Geometry: see drawing. Coordinates: mm, zero at the bounding-box minimum. A direction names the side the tool comes from. Round coordinates to 2 decimals unless told otherwise and drop trailing zeros. Loops run counter-clockwise (first coordinate to the right, second up) from the corner with the lowest first, then second, coordinate; pieces in that order, holes last. Notation, with made-up numbers: (9, 48) -> (62, 48) arc R20 ccw to (62, 76) -> close; hole circle Ø5 at (61, 60). An arc over 180 degrees is marked (long way). Write item = value, one per line.
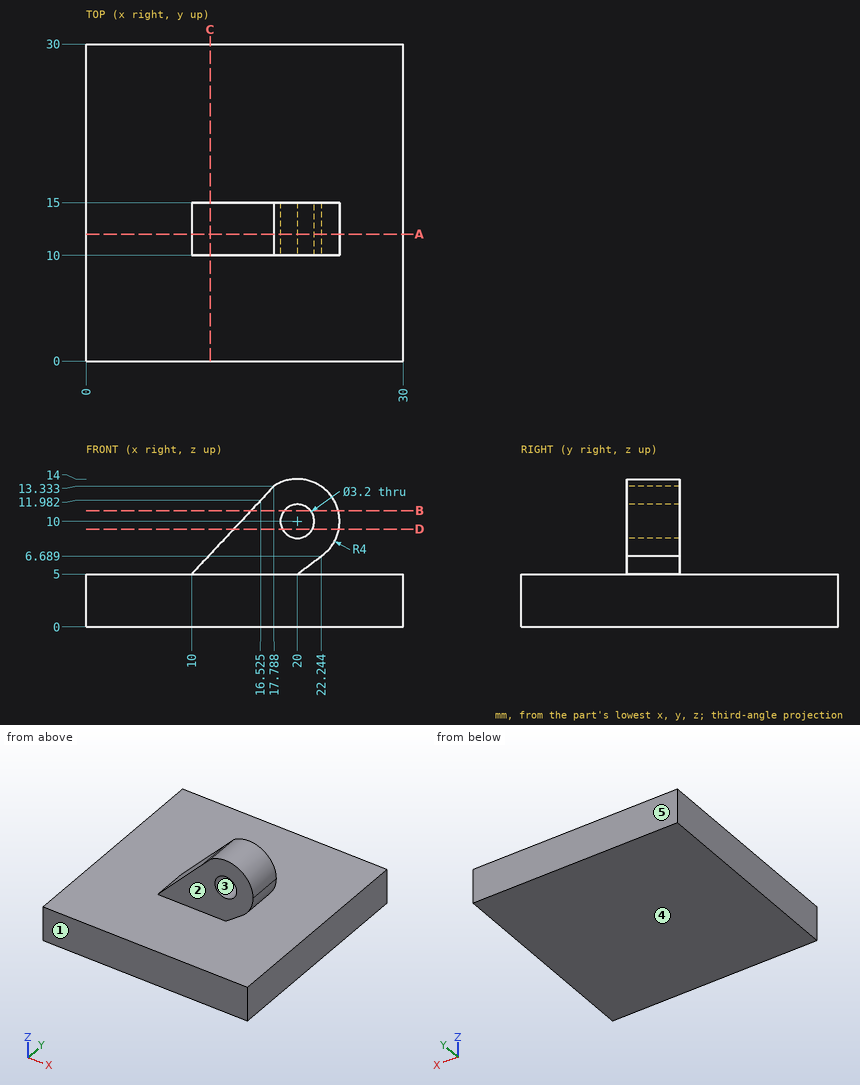
1. Section query B-B (z = 11). Return the cut outline in (x, y).
Evaluation:
outline = (15.61, 10) -> (18.75, 10) -> (18.75, 15) -> (15.61, 15) -> close; (21.25, 10) -> (23.87, 10) -> (23.87, 15) -> (21.25, 15) -> close
2. Section query A-A (y = 12). Return the cut outline in (x, z) (1 decimal).
Evaluation:
outline = (0, 0) -> (30, 0) -> (30, 5) -> (20, 5) -> (22.2, 6.7) arc R4 ccw to (24, 10) arc R4 ccw to (17.8, 13.3) -> (10, 5) -> (0, 5) -> close; hole circle Ø3.2 at (20, 10)
3. Section query D-D (z = 9.25). Return the cut outline in (x, y).
Evaluation:
outline = (13.97, 10) -> (18.59, 10) -> (18.59, 15) -> (13.97, 15) -> close; (21.41, 10) -> (23.93, 10) -> (23.93, 15) -> (21.41, 15) -> close
4. Contact query for flat-ended pins moving along their axis: pin 1 Ø4.5 at (x, z) = (19, 8.5) entering from +Y; pin 2 Ø15 at (x, y) = (15.5, 21.5) entering from +Z; pin 3 Ø6 at (y, z) = (18.5, 2.5) entering from -X; pin 4 Ø7 at (x, z) = (19, 10) entering from -Y. Output: stop coordinate, or through.
Evaluation:
pin_1 = 15
pin_2 = 13.93
pin_3 = 0
pin_4 = 10
5. Mould query, pull axis Z, two halves, no side actions, for the marked faces 3, 4 and 5. Classes: released by +Z, released by -Z, zero draft, split by the parting line, or undercut.
Evaluation:
face_3 = undercut
face_4 = released by -Z
face_5 = zero draft
6. Line query: probe 1 along Z at (x, y) = (8.25, 25.5); probe 2 along Y at (x, z) = (22.75, 11.25). Output: solid intervals per line, ascending. Write a range as from..to.
Evaluation:
probe_1 = 0..5
probe_2 = 10..15
7. Section query C-C (x = 11.75). Return the cut outline in (y, z), then the cut area to 3 significant figures.
Evaluation:
outline = (0, 0) -> (30, 0) -> (30, 5) -> (15, 5) -> (15, 6.87) -> (10, 6.87) -> (10, 5) -> (0, 5) -> close
area = 159 mm²
8. Set-up query: the marked faces 1 and 2. Return all of +Z, -Z, +X, -X, +Y, -Y with unobstructed straight access to the full face (end or side cutting, diameter ignored); none if empty.
Evaluation:
face_1 = +Z, -Z, +X, -X, -Y
face_2 = +Z, +X, -X, -Y
